The listing builds one solid part. Answer for the finished solid, in the listing's coordinates (mm). Face numbers are marked on the shaded views. Round coordinates to 2 decimals unless told otherwise and drop trailing zeros. Loops run counter-clockwise (first coordinate to the right, second up) from the corner with the lowest first, then second, coordinate; pieces in that order, holes last. Notation, with made-up numbers: M 7.25,52 L 15.25,52 A19 ccw 15.25,72 Z; hole C 9.5,-27.75 d9. An arc over 180 degrees is marked long. Answer as a JSON object with one key per item and string values.
```python
from build123d import *

# Parameters (mm, degrees)
BOSS_EXTRUDE1_DEPTH = 12.5
CUT_EXTRUDE1_DEPTH  = 1
SKETCH3_W           = 0.5
SKETCH3_H           = 2.8
CUT_EXTRUDE2_DEPTH  = 20
FILLET1_R           = 0.25
FILLET2_R           = 0.25
SKETCH4_R           = 0.4
BOSS_EXTRUDE2_DEPTH = 2.1


with BuildPart() as part:
    # Sketch1 → Boss-Extrude1 (new body)
    with BuildSketch(Plane.XY):
        with BuildLine():
            Line((-5.75, 6), (5.75, 6))
            ThreePointArc((5.75, 6), (5.926776695, 5.926776695), (6, 5.75))
            Line((6, 5.75), (6, -5.75))
            ThreePointArc((6, -5.75), (5.926776695, -5.926776695), (5.75, -6))
            Line((5.75, -6), (-5.75, -6))
            ThreePointArc((-5.75, -6), (-5.926776695, -5.926776695), (-6, -5.75))
            Line((-6, -5.75), (-6, 5.75))
            ThreePointArc((-6, 5.75), (-5.926776695, 5.926776695), (-5.75, 6))
        make_face()
    extrude(amount=BOSS_EXTRUDE1_DEPTH)

    # Sketch2 → Cut-Extrude1 (cut)
    with BuildSketch(Plane(origin=(0, 0, 0), x_dir=(-1, 0, 0), z_dir=(0, 0, -1))):
        with BuildLine():
            Line((5.25, -5.5), (-5.25, -5.5))
            ThreePointArc((-5.25, -5.5), (-5.426776695, -5.426776695), (-5.5, -5.25))
            Line((-5.5, -5.25), (-5.5, 5.25))
            ThreePointArc((-5.5, 5.25), (-5.426776695, 5.426776695), (-5.25, 5.5))
            Line((-5.25, 5.5), (5.25, 5.5))
            ThreePointArc((5.25, 5.5), (5.426776695, 5.426776695), (5.5, 5.25))
            Line((5.5, 5.25), (5.5, -5.25))
            ThreePointArc((5.5, -5.25), (5.426776695, -5.426776695), (5.25, -5.5))
        make_face()
    extrude(amount=-CUT_EXTRUDE1_DEPTH, mode=Mode.SUBTRACT)

    # Sketch3 → Cut-Extrude2 (cut)
    with BuildSketch(Plane(origin=(6, 0, 0), x_dir=(0, 0, -1), z_dir=(1, 0, 0))):
        with Locations((-0.25, 0)):
            Rectangle(SKETCH3_W, SKETCH3_H)
        with Locations((-0.25, 4.6)):
            Rectangle(SKETCH3_W, SKETCH3_H)
        with Locations((-0.25, -4.6)):
            Rectangle(SKETCH3_W, SKETCH3_H)
    extrude(amount=-CUT_EXTRUDE2_DEPTH, mode=Mode.SUBTRACT)

    # Fillet1
    fillet1_edges = [part.edges().sort_by_distance(p)[0] for p in [
        (-5.426776695, -5.426776695, 1),
        (0, -5.5, 1),
        (5.426776695, -5.426776695, 1),
        (5.5, 0, 1),
        (5.426776695, 5.426776695, 1),
        (0, 5.5, 1),
        (-5.426776695, 5.426776695, 1),
        (-5.5, 0, 1),
    ]]
    fillet(fillet1_edges, radius=FILLET1_R)

    # Fillet2
    fillet2_edges = [part.edges().sort_by_distance(p)[0] for p in [
        (5.926776695, -5.926776695, 12.5),
        (6, 0, 12.5),
        (5.926776695, 5.926776695, 12.5),
        (0, 6, 12.5),
        (-5.926776695, 5.926776695, 12.5),
        (-6, 0, 12.5),
        (-5.926776695, -5.926776695, 12.5),
        (0, -6, 12.5),
    ]]
    fillet(fillet2_edges, radius=FILLET2_R)

    # Sketch4 → Boss-Extrude2 (add)
    with BuildSketch(Plane(origin=(0, 0, 1), x_dir=(-1, 0, 0), z_dir=(0, 0, -1))):
        with Locations(Location((-5.08, 5.08, 0), (0, 0, 154.849335249))):
            Circle(SKETCH4_R)
        with Locations(Location((5.08, -5.08, 0), (0, 0, 205.150663413))):
            Circle(SKETCH4_R)
    extrude(amount=BOSS_EXTRUDE2_DEPTH)


solid = part.part
```
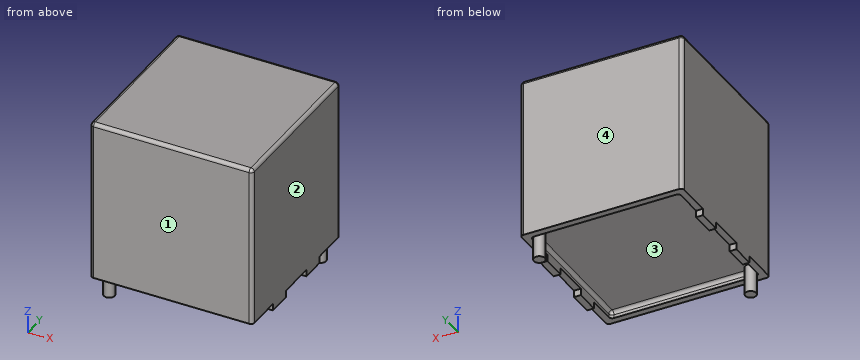
Item 1: Straight lines are drawn through the part: line 1 (Z direction, x = 1.75, y = -0.25); line 2 (Y direction, x = -5, z = -0.25). For each, find the intervals that lie inside material, in ascending order.
Values follow:
{"line 1": "1 to 12.5", "line 2": "-5.47 to -4.69"}
Item 2: Flat-ended cylindrical pins translate along their axes: P1, Ø0.6, axis at x = -6, z = 0, coming from the +Y side; P2, Ø0.6, axis at x = -5.5, y = -2.5, coming from the -Z side; P3, Ø2, axis at x = 1.5, y = 4, coming from the -Z side. Find the tip coordinate at first contact, or state that the pin passes through.
Values follow:
{"P1": "y = 3.2", "P2": "z = 0", "P3": "z = 1"}
Item 3: The part is cut by section A-A (x = -4.25). Give the vertices of the cut face in (y, z), then the cut area to 4 significant figures.
Values follow:
{"outline": "M -6,0.5 L -5.5,0.5 L -5.5,0.75 A0.25 cw -5.25,1 L 5.25,1 A0.25 cw 5.5,0.75 L 5.5,0.5 L 6,0.5 L 6,12.25 A0.25 ccw 5.75,12.5 L -5.75,12.5 A0.25 ccw -6,12.25 Z", "area": "138.5 mm^2"}
Item 4: Determine the mould class of the marked faces 1, 2, 3 and 4 for opening direction Y: released by +Y, released by -Y, zero draft, split by the parting line, or undercut.
Values follow:
{"face 1": "released by -Y", "face 2": "zero draft", "face 3": "undercut", "face 4": "released by +Y"}
